Autodesk Inventor part; units mm, degrees
ref_plane "Work Plane3" through (0, 0, 225) normal (0, 0, 1) x (1, 0, 0)
ref_plane "YZ Plane" through (0, 0, 0) normal (1, 0, 0) x (0, 1, 0)
ref_plane "XZ Plane" through (0, 0, 0) normal (0, 1, 0) x (-1, 0, 0)
sketch "Sketch1" plane through (0, 0, 0) normal (0, 0, 1) x (1, 0, 0)
  line L0 (-197.9412, -291.7647) -> (-197.9412, 108.2353)
  line L1 (-197.9412, 108.2353) -> (-97.9412, 108.2353)
  line L2 (-97.9412, 108.2353) -> (-97.9412, 258.2353)
  line L3 (-97.9412, 258.2353) -> (-22.9412, 258.2353)
  line L4 (-22.9412, 258.2353) -> (-22.9412, 195.8824)
  line L5 (-22.9412, 195.8824) -> (127.0588, 195.8824)
  line L6 (127.0588, 195.8824) -> (127.0588, 258.2353)
  line L7 (127.0588, 258.2353) -> (302.0588, 258.2353)
  line L8 (302.0588, 258.2353) -> (302.0588, -291.7647)
  line L9 (302.0588, -291.7647) -> (-197.9412, -291.7647)
  point P0 (0, 0)
  dimension "d0" = 100
  dimension "d1" = 75
  dimension "d2" = 150
  dimension "d3" = 500
  dimension "d4" = 400
  dimension "d5" = 550
extrude "Extrusion1" add sketch "Sketch1" along normal blind 75
sketch "Sketch2" plane through (0, 0, 75) normal (0, 0, 1) x (1, 0, 0)
  point P0 (0, 0)
ref_plane "Work Plane1" through (0, 0, 75) normal (0, 0, 1) x (1, 0, 0)
sketch "Sketch3" plane through (0, 0, 75) normal (0, 0, 1) x (1, 0, 0)
  line L0 (-197.9412, -291.7647) -> (-197.9412, 8.2353)
  line L1 (-197.9412, 8.2353) -> (302.0588, 8.2353)
  line L2 (302.0588, 8.2353) -> (302.0588, -291.7647)
  line L3 (302.0588, -291.7647) -> (-197.9412, -291.7647)
  line L4 (-197.9412, -291.7647) -> (302.0588, -291.7647)
  line L5 (-197.9412, 108.2353) -> (-197.9412, -291.7647)
  point P0 (0, 0)
  dimension "d9" = 300
  dimension "d10" = 500
extrude "Extrusion2" add sketch "Sketch3" along normal blind 75
ref_plane "Work Plane2" through (0, 0, 150) normal (0, 0, 1) x (1, 0, 0)
sketch "Sketch4" plane through (0, 0, 150) normal (0, 0, 1) x (1, 0, 0)
  line L0 (-197.9412, 108.2353) -> (-197.9412, -291.7647)
  line L1 (-197.9412, -191.7647) -> (302.0588, -191.7647)
  line L2 (302.0588, -291.7647) -> (302.0588, 258.2353)
  line L3 (-197.9412, -291.7647) -> (302.0588, -291.7647)
  point P0 (0, 0)
  dimension "d14" = 100
extrude "Extrusion3" add sketch "Sketch4" along normal blind 75
ref_plane "Work Plane3" through (0, 0, 225) normal (0, 0, 1) x (1, 0, 0)
sketch "Sketch5" plane through (0, 0, 225) normal (0, 0, 1) x (1, 0, 0)
  line L0 (-197.9412, 8.2353) -> (-197.9412, -191.7647)
  line L1 (-197.9412, -91.7647) -> (2.0588, -91.7647)
  line L2 (2.0588, -91.7647) -> (2.0588, -191.7647)
  line L3 (-197.9412, -191.7647) -> (302.0588, -191.7647)
  line L4 (102.0588, -191.7647) -> (102.0588, -91.7647)
  line L5 (102.0588, -91.7647) -> (302.0588, -91.7647)
  line L6 (302.0588, -191.7647) -> (-197.9412, -191.7647)
  line L7 (302.0588, -91.7647) -> (302.0588, -191.7647)
  line L8 (302.0588, -191.7647) -> (302.0588, -291.7647)
  line L9 (-197.9412, -291.7647) -> (302.0588, -291.7647)
  line L10 (302.0588, -291.7647) -> (-197.9412, -291.7647)
  line L11 (-197.9412, -291.7647) -> (-197.9412, -91.7647)
  line L12 (2.0588, -191.7647) -> (102.0588, -191.7647)
  point P0 (0, 0)
  dimension "d18" = 200
  dimension "d19" = 200
  dimension "d20" = 100
  dimension "d21" = 100
extrude "Extrusion4" add sketch "Sketch5" along normal blind 75
properties part number "BT011"
CAD build for the part. Positions are in the model's coordinates, mm. A direction names the side the tool comes from. Round coordinates to 2 decimals unless told otherwise and drop trailing zeros. Loops run counter-clockwise (first coordinate to the right, second up) from the corner with the lowest first, then second, coordinate; pieces in that order, holes last. Notation, with made-up numbers: M -17.75,-26 L 10.25,-26 A13 ccw 10.25,-9 Z; hole C 41.25,57 d7. An arc over 180 degrees is marked long. One line per question, with ' | ' between items. Start each with the question number.
Item 1: Which spindle directions (+Z, -Z, +X, -X, +Y, -Y) get a long thin tool onto all of the face, cutting with end or side? Do faces 1 (the flat face through (2.059, -141, 262)), 2 (the flat face through (-97.941, 182, 37)), 3 (the flat face through (127.059, 227, 37)), 4 (the flat face through (49, 8.235, 112)), 5 (the flat face through (201, -141, 225)). Say none if no direction does.
Item 2: Cut at B-B, the plane x = 235. Write the cut outline in (y, z), plus the area to 4 significant figures.
Item 3: Two-plate mould, pull along Z, no slides. Class faces 6 (the flat face through (104, 107, 75)), 7 (the flat face through (51, 195.882, 37)), 8 (the flat face through (49, -191.765, 191)): pulls with the +Z half, pulls with the -Z half, needs draft (parallel to the pull), parting line crosses it, or undercut.
Item 4: Cut at A-A, the plane y = -102.5. Write the cut outline in (x, z), plus the area to 3 significant figures.
Item 5: Pin check, flat tips, straight feed: pin 1 Ø18.5 at (y, z) = (225.5, 49.5) entering from -X; pin 2 Ø1.5 at (x, z) = (216, 136) entering from +Y. Stop position of each tip, or through.
Item 6: Cut at D-D, the plane y = 145.5. Write the cut outline in (x, z).
Item 7: Wall check: line 1 (Z direction, x = 272.5, y = -146.5); line 2 (Y direction, x = 134, z = 240.5); line 3 (Y direction, x = 28.5, z = 92). Give the ranges that are in metal, low to high.
Item 8: Cut at C-C, the plane z = 276. Write the cut outline in (x, y), plus the area to 3 significant figures.
Responses:
1) face 1: +Z, +Y | face 2: +Z, -Z, -X, +Y | face 3: +Z, -Z, +Y | face 4: +Z, +X, -X, +Y | face 5: +X, -X, +Y
2) outline: M -291.76,0 L 258.24,0 L 258.24,75 L 8.24,75 L 8.24,150 L -191.76,150 L -191.76,225 L -91.76,225 L -91.76,300 L -291.76,300 Z | area: 86,250 mm²
3) face 6: pulls with the +Z half | face 7: needs draft | face 8: undercut
4) outline: M -197.94,0 L 302.06,0 L 302.06,150 L -197.94,150 Z; M -197.94,225 L 2.06,225 L 2.06,300 L -197.94,300 Z; M 102.06,225 L 302.06,225 L 302.06,300 L 102.06,300 Z | area: 105,000 mm²
5) pin 1: stops at x = -97.94 | pin 2: stops at y = 8.24
6) outline: M -97.94,0 L 302.06,0 L 302.06,75 L -97.94,75 Z
7) line 1: z = 0 to 150, 225 to 300 | line 2: y = -291.76 to -91.76 | line 3: y = -291.76 to 8.24
8) outline: M -197.94,-291.76 L 302.06,-291.76 L 302.06,-91.76 L 102.06,-91.76 L 102.06,-191.76 L 2.06,-191.76 L 2.06,-91.76 L -197.94,-91.76 Z | area: 90,000 mm²
